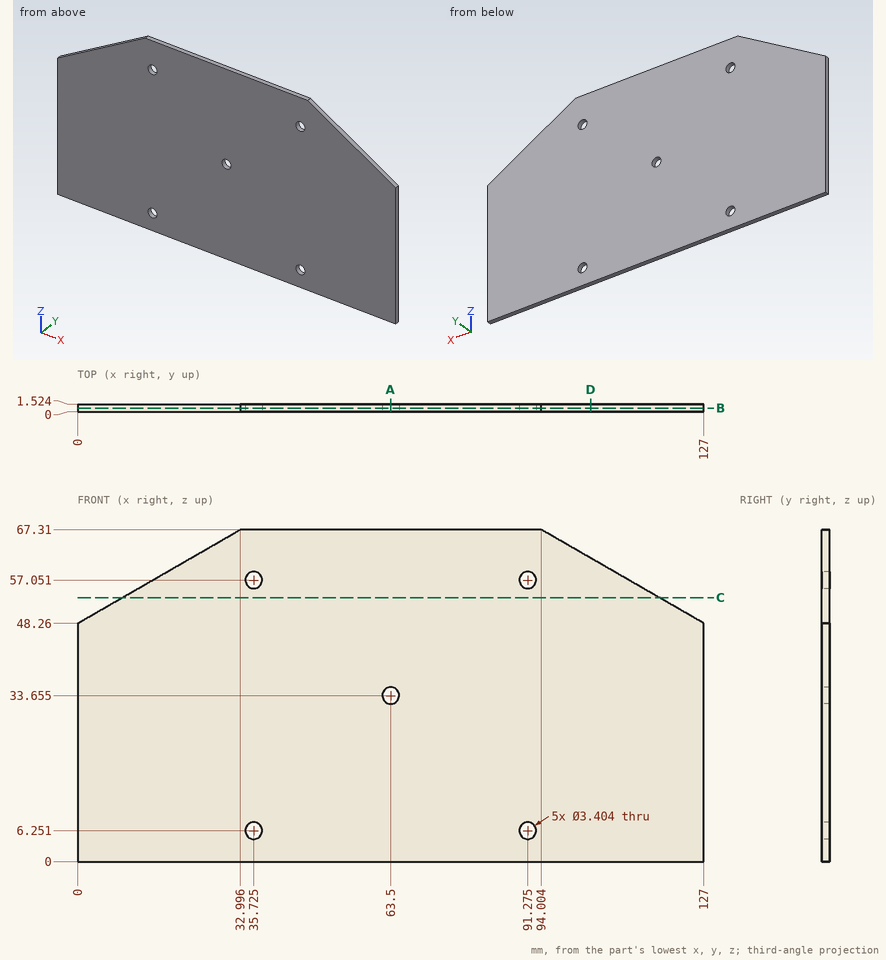
Answer from the drawing. Dimensions are ordinates in mm from the lowest x, y and z of the part. Give positions to 0.01 mm unless a question says otherwise; leave off trailing zeros. Write each loop counter-clockwise with the first axis right and the second up, starting at its lowest first coordinate (ties: lowest second). Pieces come first, ordered by that corner, then holes.
1) Section D-D (x = 104) is taken. Write down the section's boundary in (y, z).
2) Section B-B (y = 0.7) is taken. Count the separate pieces of the cut face and the enclosed holes in it, and give its area (3 significant figures).
3) Find the intervals of material crossed by L1, parallel to X at y = 1.2, z = 56.5 (1 decimal); L2, parallel to Z at x = 90, y = 0.25 (1 decimal); L3, parallel to X at y = 0.95, z = 56 (1 decimal), in increasing order.
4) Given P1, Ø4.5, axis at x = 91.27, z = 6.25, coming from the +Y side, flat-ended and moving along its own axis, determine where the tip first touches the part or whether it passes through.
5) Section A-A (x = 63.5) is taken. Write down the section's boundary in (y, z).
6) Section C-C (z = 53.5) is taken. Write down the section's boundary in (x, y).
Response:
1. outline: (0, 0) - (1.52, 0) - (1.52, 61.54) - (0, 61.54) - close
2. separate pieces: 1
2. enclosed holes: 5
2. area: 7,870 mm2
3. L1: x = 14.3 to 34.1, 37.3 to 89.7, 92.9 to 112.7
3. L2: z = 0 to 5.1, 7.4 to 55.9, 58.2 to 67.3
3. L3: x = 13.4 to 34.4, 37.1 to 89.9, 92.6 to 113.6
4. P1: stops at y = 1.52
5. outline: (0, 0) - (1.52, 0) - (1.52, 31.95) - (0, 31.95) - close; (0, 35.36) - (1.52, 35.36) - (1.52, 67.31) - (0, 67.31) - close
6. outline: (9.08, 0) - (117.92, 0) - (117.92, 1.52) - (9.08, 1.52) - close
